The drawing under review shows one solid part. Ordinate dimensions are in mm from its lowest x, y, z. A direction names the side the tool comes from. Coordinates: 2 decimals unless noted, no trailing zeros. Write each loop counter-clockwise with the first axis right and the second up, starting at its lowest first coordinate (ties: lowest second). Pieces come first, ordered by that corner, then holes.
1) Insertion check: P1, Ø10, axis at x = 9.5, y = 12.5, coming from the +Z side; P2, Ø4, axis at x = 8, y = 12, coming from the -Z side; P3, Ø6, axis at y = 8.5, z = 17, coming from the +X side. Each pin has a flat end and moves straight along its axis. Give the tip position at first contact, or say it passes through.
2) We need section A-A on y = 18. Write out the cut boundary in (x, z).
3) We need section D-D on y = 12. Write out the cut boundary in (x, z).
4) For the marked faces 1, 2 and 3, list the 3-axis set-ups (+Z, -Z, +X, -X, +Y, -Y) from which the entire face can be reached by the end or side of a thin tool; tool diameter is ignored.
5) We need section B-B on z = 15. Write out the cut boundary in (x, y), then the cut area to 3 significant figures.
6) We need section C-C on x = 7.5. Write out the cut boundary in (y, z).
7) To check wall thickness, follow line 1 along Y through (x, z) = (8, 10.4); line 2 along X through (y, z) = (14.5, 17.75); line 3 along Z through (x, y) = (20.25, 7). State the ranges of each line that lie inside material, in increasing order.
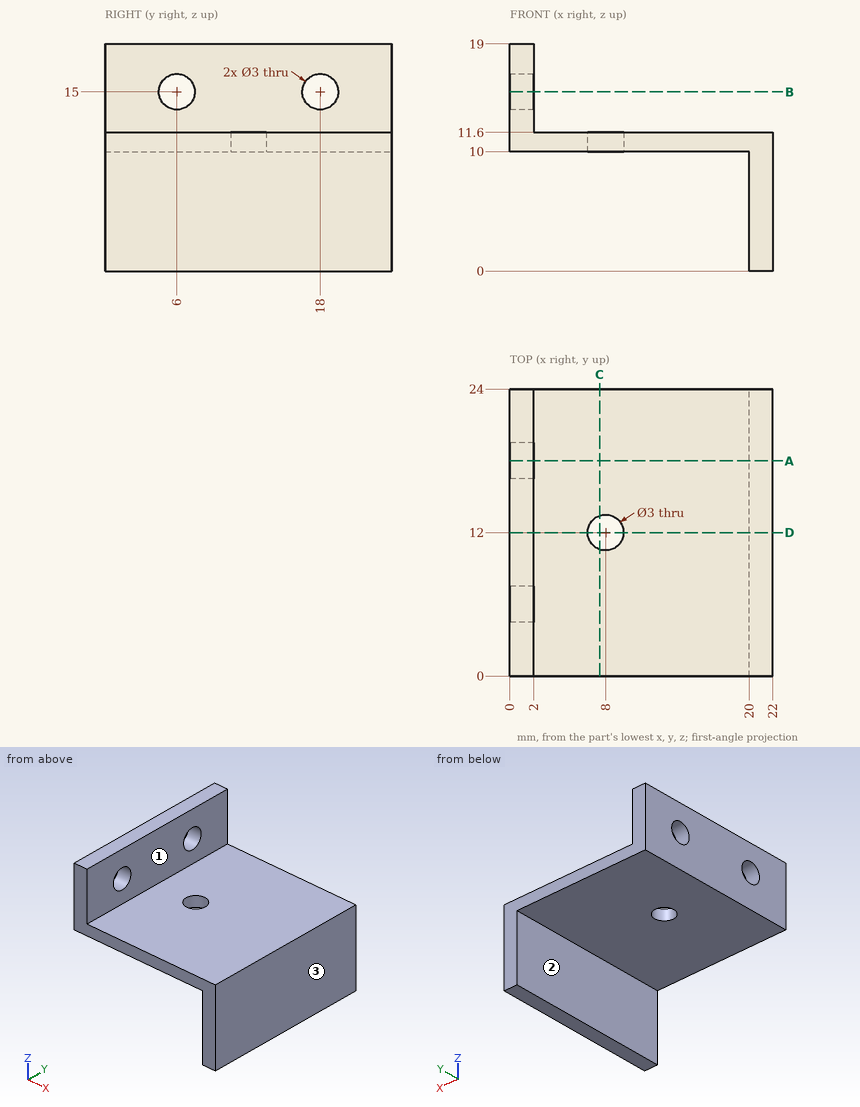
Result:
1. P1: stops at z = 11.6
1. P2: stops at z = 10
1. P3: stops at x = 2
2. outline: (0, 10) - (20, 10) - (20, 0) - (22, 0) - (22, 11.6) - (2, 11.6) - (2, 13.5) - (0, 13.5) - close; (0, 16.5) - (2, 16.5) - (2, 19) - (0, 19) - close
3. outline: (0, 10) - (6.5, 10) - (6.5, 11.6) - (2, 11.6) - (2, 19) - (0, 19) - close; (9.5, 10) - (20, 10) - (20, 0) - (22, 0) - (22, 11.6) - (9.5, 11.6) - close
4. face 1: +Z, +X, +Y, -Y
4. face 2: -Z, -X, +Y, -Y
4. face 3: +Z, -Z, +X, +Y, -Y
5. outline: (0, 0) - (2, 0) - (2, 4.5) - (0, 4.5) - close; (0, 7.5) - (2, 7.5) - (2, 16.5) - (0, 16.5) - close; (0, 19.5) - (2, 19.5) - (2, 24) - (0, 24) - close
5. area: 36.0 mm2
6. outline: (0, 10) - (10.59, 10) - (10.59, 11.6) - (0, 11.6) - close; (13.41, 10) - (24, 10) - (24, 11.6) - (13.41, 11.6) - close
7. line 1: y = 0 to 10.5, 13.5 to 24
7. line 2: x = 0 to 2
7. line 3: z = 0 to 11.6
